Check sheet for the modelled part. Datum: model origin and axes. Units: mm. A direction names the side the tool comes from. Round coordinates to 2 decimals unless told otherwise and drop trailing zeros. Order: outer loops, then holes, each group sorted by start corner. A loop starts at its lowest first (then second) coordinate and runs counter-clockwise, first axis right, second up.
Q1. Mould release check, pull along Y, two halves, no side actions. Record for faces 1 (the flat face through (-54, 27.416, 12)), 2 (the flat face through (-51, 46, 0)), 3 (the flat face through (-52, 29.916, 11)): +Y half, -Y half, draft (parallel to the pull), parting line (faces both ways), or undercut.
Q2. Depth check by flat-ended pin: P1, Ø1.5, axis at y = 32, z = 18, coming from the -X side; P2, Ø1.5, axis at x = -42.5, y = 36, coming from the -Z side; P3, Ø10, axis at y = 36.5, z = 7, coming from the -X side. Enter the tip coordinate at first touch or a pass-through.
Q3. Set-up check for faces 4 (the flat face through (-51, 47.416, 12)), 5 (the flat face through (-51, 44.916, 11)): record each of +Z, -Z, +X, -X, +Y, -Y from which the full face is reachable in a straight line by a thin tool's end or side.
Q4. Cross-section at B-B on z = 10.5. Record the cut outline in (x, y), then the cut area to 3 significant figures.
Q5. Cross-section at C-C on y = 35.5. Record the cut outline in (x, z).
Q6. Scan lines: probe 1 along Y at (x, z) = (-54.75, 8.75); probe 2 along Z at (x, y) = (-57.5, 30); probe 3 along X at (y, z) = (32.75, 11). Record each from-to range of solid material in increasing order.
Q7. Cross-section at D-D on y = 29.25. Record the cut outline in (x, z), then the cut area to 3 significant figures.
Q8. Cross-section at A-A on x = -58. Record the cut outline in (y, z).
from build123d import *

# Parameters (mm, degrees)
F1_DEPTH = 25
F2_R     = 5
F3_T     = -2.5


with BuildPart() as f1:
    # F0 (on Top) → F1 (new body)
    with BuildSketch(Plane.XY):
        Polygon((-39.500976, 47.416381), (-63.099665, 47.416381), (-62.593336, 27.416381), (-39.500976, 27.416381), align=None)
    extrude(amount=F1_DEPTH)

    # F2
    f2_edges = [f1.edges().sort_by_distance(p)[0] for p in [
        (-39.500976, 27.416381, 12.5),
    ]]
    fillet(f2_edges, radius=F2_R)

    # F3
    f3_openings = [f1.faces().sort_by_distance(p)[0] for p in [
        (-51.296904, 37.556207, 0),
    ]]
    offset(amount=F3_T, openings=f3_openings)


solid = f1.part
Results found:
1. face 1: -Y half
1. face 2: draft
1. face 3: undercut
2. P1: stops at x = -62.73
2. P2: stops at z = 0
2. P3: stops at x = -62.95
3. face 4: +Z, -Z, +X, -X, +Y
3. face 5: -Z
4. outline: (-63.1, 47.42) - (-62.59, 27.42) - (-44.5, 27.42) arc R5 ccw to (-39.5, 32.42) - (-39.5, 47.42) - close; hole (-60.54, 44.92) - (-60.16, 29.92) - (-44.5, 29.92) arc R2.5 ccw to (-42, 32.42) - (-42, 44.92) - close
4. area: 188 mm2
5. outline: (-62.8, 0) - (-60.3, 0) - (-60.3, 22.5) - (-42, 22.5) - (-42, 0) - (-39.5, 0) - (-39.5, 25) - (-62.8, 25) - close
6. probe 1: y = 27.42 to 29.92, 44.92 to 47.42
6. probe 2: z = 22.5 to 25
6. probe 3: x = -62.73 to -60.23, -42 to -39.5
7. outline: (-62.64, 0) - (-40.63, 0) - (-40.63, 25) - (-62.64, 25) - close
7. area: 550 mm2
8. outline: (27.42, 0) - (29.92, 0) - (29.92, 22.5) - (44.92, 22.5) - (44.92, 0) - (47.42, 0) - (47.42, 25) - (27.42, 25) - close
